Design review of the part shown in the three views and the two pictorial views. Dimensions are in mm from the part's minimum x, y and z. A direction names the side the tool comes from. Give positions to 0.01 mm unless a question says otherwise; leave off trailing zeros. Loops run counter-clockwise (first coordinate to the right, second up) from the corner with the lowest first, then second, coordinate; pieces in that order, holes last. Notation, with made-up numbers: (31, 54) - (65, 54) arc R17 ccw to (65, 72) - close; hole circle Ø2 at (66, 17.5). An arc over 180 degrees is marked (long way). Answer in a Markdown table with one row per item.
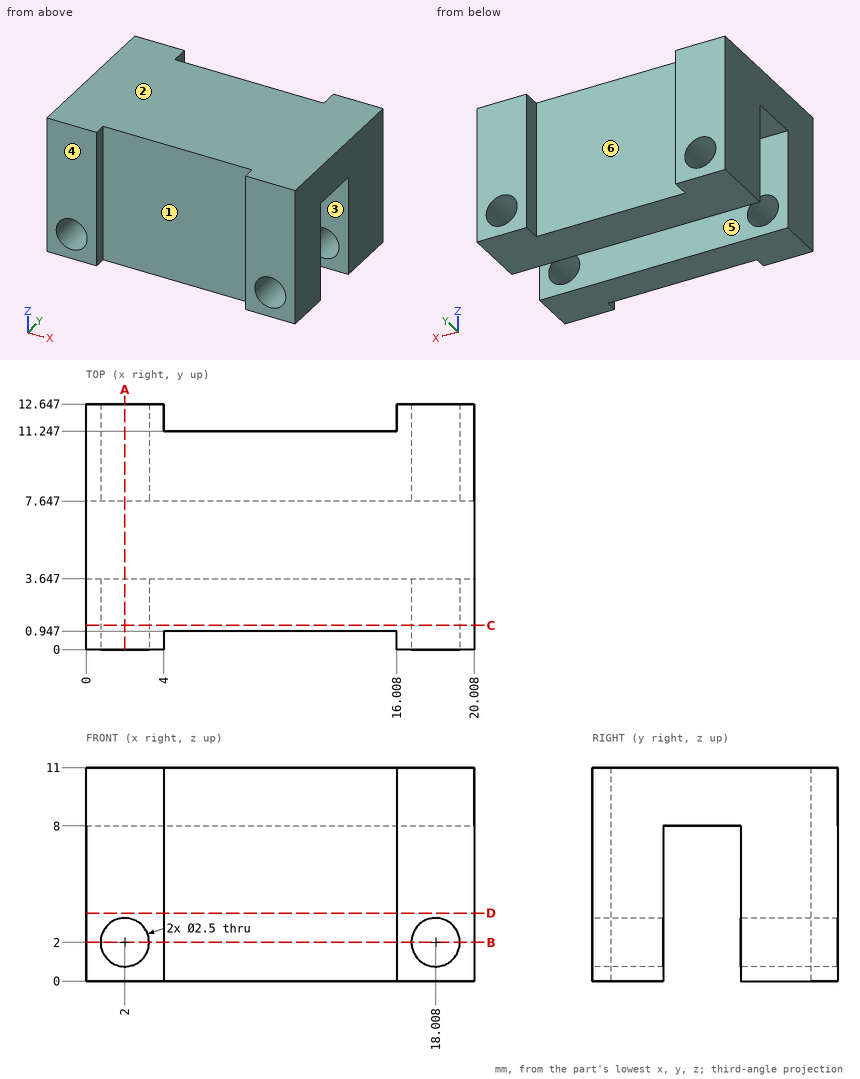
1. Clearance check with flat-ended pins moving along their axes: pin 1 (3.5 mm diameter, centred on x = 11, z = 3, fed in from -Y); pin 2 (4 mm diameter, centred on x = 7, z = 4.5, fed in from +Y); pin 3 (1.2 mm diameter, centred on x = 13.5, y = 5.5, fed in from -Z). State where each tip first meets the part, or that it passes through.
Values:
| item | result |
|---|---|
| pin 1 | stops at y = 0.95 |
| pin 2 | stops at y = 11.25 |
| pin 3 | stops at z = 8 |
2. We need section C-C, the plane y = 1.25. Give the boundary of the cut face in (x, z), and give its area (3 significant figures).
Values:
| item | result |
|---|---|
| outline | (0, 0) - (20.01, 0) - (20.01, 11) - (0, 11) - close; hole circle Ø2.5 at (2, 2); hole circle Ø2.5 at (18.01, 2) |
| area | 210 mm^2 |
3. Mouldability with a two-part tool opening along Y and no side actions: class the marked faces 4, 5 and 6 as released by +Y, released by -Y, zero draft, split by the parting line, or undercut.
Values:
| item | result |
|---|---|
| face 4 | released by -Y |
| face 5 | undercut |
| face 6 | released by +Y |
4. We need section D-D, the plane z = 3.5. Give the boundary of the cut face in (x, y), and give its area (3 significant figures).
Values:
| item | result |
|---|---|
| outline | (0, 0) - (4, 0) - (4, 0.95) - (16.01, 0.95) - (16.01, 0) - (20.01, 0) - (20.01, 3.65) - (0, 3.65) - close; (0, 7.65) - (20.01, 7.65) - (20.01, 12.65) - (16.01, 12.65) - (16.01, 11.25) - (4, 11.25) - (4, 12.65) - (0, 12.65) - close |
| area | 145 mm^2 |
5. For the marked faces 1, 2 and 3, list the 3-axis set-ups (+Z, -Z, +X, -X, +Y, -Y) from which the entire face can be reached by the end or side of a thin tool; tool diameter is ignored.
Values:
| item | result |
|---|---|
| face 1 | +Z, -Z, -Y |
| face 2 | +Z, +X, -X, +Y, -Y |
| face 3 | -Z, +X, -X |
6. We need section A-A, the plane x = 2. Give the boundary of the cut face in (y, z).
Values:
| item | result |
|---|---|
| outline | (0, 0) - (3.65, 0) - (3.65, 0.75) - (0, 0.75) - close; (0, 3.25) - (3.65, 3.25) - (3.65, 8) - (7.65, 8) - (7.65, 3.25) - (12.65, 3.25) - (12.65, 11) - (0, 11) - close; (7.65, 0) - (12.65, 0) - (12.65, 0.75) - (7.65, 0.75) - close |
7. Wall thickness on line 1 (X direction, y = 11.15, z = 2); line 2 (Y direction, x = 10, z = 5.25); line 3 (Z direction, x = 2, y = 2.4): over which ranges is each line inside the solid? List them lowest first. Write a range as [from, to].
Values:
| item | result |
|---|---|
| line 1 | x = [0, 0.75], [3.25, 16.76], [19.26, 20.01] |
| line 2 | y = [0.95, 3.65], [7.65, 11.25] |
| line 3 | z = [0, 0.75], [3.25, 11] |
8. We need section B-B, the plane z = 2. Count the separate pieces of the cut face and the enclosed holes in it.
Values:
| item | result |
|---|---|
| separate pieces | 6 |
| enclosed holes | 0 |
